Build history of the part. All positions in model axes, mm. A direction names the side the tool comes from. Round coordinates to 2 decimals unless told otherwise and drop trailing zeros. Write each loop counter-clockwise with the first axis right and the second up, starting at its lowest first coordinate (ties: lowest second). Pieces come first, ordered by that corner, then holes.
from build123d import *

# Parameters (mm, degrees)
SKETCH1_W           = 250
SKETCH1_H           = 150
BOSS_EXTRUDE1_DEPTH = 20
FILLET1_R           = 12.7
FILLET2_R           = 9.5
CAVITY1_START       = -65
CAVITY1_OUTLINE_W   = 20
CAVITY1_OUTLINE_H   = 5.4
CAVITY1_DEPTH       = 130
CAVITY1_START_2     = -2.7
CAVITY1_2_OUTLINE_W = 20
CAVITY1_2_OUTLINE_H = 33.9
CAVITY1_2_DEPTH     = 5.4


# Read off the part's stored shape, not the designer's step: Cavity1
with BuildPart() as part:
    # Sketch1 → Boss-Extrude1 (new body)
    with BuildSketch(Plane(origin=(0, 0, 0), x_dir=(1, 0, 0), z_dir=(0, 1, 0))):
        Rectangle(SKETCH1_W, SKETCH1_H)
    extrude(amount=-BOSS_EXTRUDE1_DEPTH)

    # Fillet1
    fillet1_edges = [part.edges().sort_by_distance(p)[0] for p in [
        (125, -10, 75),
        (-125, -10, 75),
        (-125, -10, -75),
        (125, -10, -75),
    ]]
    fillet(fillet1_edges, radius=FILLET1_R)

    # Fillet2
    fillet2_edges = [part.edges().sort_by_distance(p)[0] for p in [
        (0, 0, -75),
        (125, 0, 0),
        (-125, 0, 0),
        (0, 0, 75),
        (121.280256121, 0, 71.280256121),
        (-121.280256121, 0, 71.280256121),
        (121.280256121, 0, -71.280256121),
        (-121.280256121, 0, -71.280256121),
    ]]
    fillet(fillet2_edges, radius=FILLET2_R)

    # Cavity1 outline → Cavity1 (cut)
    with BuildSketch(Plane.YZ.offset(CAVITY1_START)):
        with Locations((-10, 19.65)):
            Rectangle(CAVITY1_OUTLINE_W, CAVITY1_OUTLINE_H)
        with Locations((-10, -19.65)):
            Rectangle(CAVITY1_OUTLINE_W, CAVITY1_OUTLINE_H)
    extrude(amount=CAVITY1_DEPTH, mode=Mode.SUBTRACT)

    # Cavity1 2 outline → Cavity1 2 (cut)
    with BuildSketch(Plane.YZ.offset(CAVITY1_START_2)):
        with Locations((-10, 0)):
            Rectangle(CAVITY1_2_OUTLINE_W, CAVITY1_2_OUTLINE_H)
        with BuildLine():
            Line((-20, 22.35), (0, 22.35))
            Line((0, 22.35), (0, 62.3))
            Line((0, 62.3), (-19, 62.3))
            ThreePointArc((-19, 62.3), (-19.707106781, 62.007106781), (-20, 61.3))
            Line((-20, 61.3), (-20, 22.35))
        make_face()
        with BuildLine():
            Line((0, -62.3), (0, -22.35))
            Line((0, -22.35), (-20, -22.35))
            Line((-20, -22.35), (-20, -61.3))
            ThreePointArc((-20, -61.3), (-19.707106781, -62.007106781), (-19, -62.3))
            Line((-19, -62.3), (0, -62.3))
        make_face()
    extrude(amount=CAVITY1_2_DEPTH, mode=Mode.SUBTRACT)


solid = part.part
1) Slice it at D-D (z = -53). Write the cut outline in (x, y).
Results:
outline: (-125, -20) - (-2.7, -20) - (-2.7, 0) - (-115.5, 0) arc R9.5 ccw to (-125, -9.5) - close; (2.7, -20) - (125, -20) - (125, -9.5) arc R9.5 ccw to (115.5, 0) - (2.7, 0) - close
2) Which spindle directions (+Z, -Z, +X, -X, +Y, -Y) get a long thin tool onto all of the face, cutting with end or side? Do faces 1 (the cylindrical face through (-121.38, -14.82, -71.18)), 2 (the flat face through (0, -10, -62.3)), 3 (the flat face through (-65, -10, 20)). Say none if no direction does.
Results:
face 1: -Z, -X, +Y, -Y
face 2: +Y
face 3: +Y, -Y
3) Wall check: L1, parallel to Z at x = -13.5, y = -17.25; L2, parallel to Z at x = 44, y = -8.5; L3, parallel to X at y = -10, z = 0. Give the ranges that are in metal, low to high.
Results:
L1: z = -75 to -22.35, -16.95 to 16.95, 22.35 to 75
L2: z = -74.95 to -22.35, -16.95 to 16.95, 22.35 to 74.95
L3: x = -125 to -2.7, 2.7 to 125
4) Pin check, flat tips, straight feed: pin 1 Ø3 at (x, y) = (-72, -8) entering from -Z; pin 2 Ø4.5 at (y, z) = (-7, 21) entering from +X; pin 3 Ø4 at (x, y) = (52.5, -7) entering from +Z; pin 4 Ø1.6 at (y, z) = (-7.5, -20) entering from -X. Stop position of each tip, or through.
Results:
pin 1: stops at z = -75
pin 2: stops at x = 125
pin 3: stops at z = 74.99
pin 4: stops at x = -124.92
5) Slice it at C-C (x = -17). Write the cut outline in (y, z), plus the area to 3 significant figures.
Results:
outline: (-20, -75) - (-9.5, -75) arc R9.5 ccw to (0, -65.5) - (0, -22.35) - (-20, -22.35) - close; (-20, -16.95) - (0, -16.95) - (0, 16.95) - (-20, 16.95) - close; (-20, 22.35) - (0, 22.35) - (0, 65.5) arc R9.5 ccw to (-9.5, 75) - (-20, 75) - close
area: 2,750 mm2
6) Slice it at A-A (z = -19.5). Write the cut outline in (x, y).
Results:
outline: (-125, -20) - (-65, -20) - (-65, 0) - (-115.5, 0) arc R9.5 ccw to (-125, -9.5) - close; (65, -20) - (125, -20) - (125, -9.5) arc R9.5 ccw to (115.5, 0) - (65, 0) - close
7) Mould opens along Z. For faces 4 (the cylindrical face through (1.572, -2.709, -72.143)), 5 (the flat face through (-27, 0, -1)), 6 (the flat face through (0, -9, 62.3)), 7 (the flat face through (33, -10, 16.95)) say: released by +Z, released by -Z, zero draft, split by the parting line, or undercut.
Results:
face 4: released by -Z
face 5: zero draft
face 6: undercut
face 7: undercut
8) Slice it at B-B (y = -14). Write the cut outline in (x, z).
Results:
outline: (-125, -62.3) arc R12.7 ccw to (-112.3, -75) - (112.3, -75) arc R12.7 ccw to (125, -62.3) - (125, 62.3) arc R12.7 ccw to (112.3, 75) - (-112.3, 75) arc R12.7 ccw to (-125, 62.3) - close; hole (-65, -22.35) - (-2.7, -22.35) - (-2.7, -62.3) - (2.7, -62.3) - (2.7, -22.35) - (65, -22.35) - (65, -16.95) - (2.7, -16.95) - (2.7, 16.95) - (65, 16.95) - (65, 22.35) - (2.7, 22.35) - (2.7, 62.3) - (-2.7, 62.3) - (-2.7, 22.35) - (-65, 22.35) - (-65, 16.95) - (-2.7, 16.95) - (-2.7, -16.95) - (-65, -16.95) - close
